CAD build for the part. Positions are in the model's coordinates, mm. A direction names the side the tool comes from. Round coordinates to 2 decimals unless told otherwise and drop trailing zeros. Loops run counter-clockwise (first coordinate to the right, second up) from the corner with the lowest first, then second, coordinate; pieces in that order, holes last. Notation, with made-up numbers: M 7,45 L 38,45 A20 ccw 38,69 Z; hole C 86,-26 d2. An arc over 180 degrees is marked long. Use one line per item in the form item = value.
Autodesk Inventor part; units mm, degrees
ref_plane "Work Plane3" through (-33.4299, 11.4299, 16.4) normal (0, 0, -1) x (0, 1, 0)
ref_plane "YZ Plane" through (0, 0, 0) normal (1, 0, 0) x (0, 1, 0)
ref_plane "XZ Plane" through (0, 0, 0) normal (0, 1, 0) x (-1, 0, 0)
ref_plane "Work Plane1" through (0, 0, 10) normal (0, 0, 1) x (1, 0, 0)
sketch "Sketch1" plane through (0, 0, 10) normal (0, 0, 1) x (1, 0, 0)
  line L0 (-4.0299, -0.3538) -> (-2.2322, 1.4439) construction
  arc A0 (-1.4439, 2.2322) -> (-2.2322, 1.4439) centre (-0.9299, 0.9299) ccw construction
  line L1 (-1.4439, 2.2322) -> (0.3538, 4.0299) construction
  line L2 (-37.8299, 42.2137) -> (-37.8299, 45.8299) construction
  line L3 (-37.8299, 45.8299) -> (-4.0299, 45.8299) construction
  line L4 (-4.0299, 45.8299) -> (-4.0299, 42.2137) construction
  line L5 (-4.0299, 4.0299) -> (0.3538, 4.0299)
  circle A1 centre (-20.9299, 20.9299) radius 17.5
  line L6 (-20.9299, 58.9723) -> (17.1124, 20.9299) construction
  line L7 (17.1124, 20.9299) -> (-20.9299, -17.1124) construction
  line L8 (-20.9299, -17.1124) -> (-58.9723, 20.9299) construction
  line L9 (-58.9723, 20.9299) -> (-20.9299, 58.9723) construction
  line L10 (-20.9299, 58.9723) -> (-20.9299, -17.1124) construction
  line L11 (17.1124, 20.9299) -> (-58.9723, 20.9299) construction
  line L12 (-20.9299, 58.9723) -> (32.8701, 58.9723) construction
  line L13 (-43.4299, 43.4299) -> (1.5701, 43.4299) construction
  line L14 (1.5701, 43.4299) -> (1.5701, -1.5701) construction
  line L15 (1.5701, -1.5701) -> (-43.4299, -1.5701) construction
  line L16 (-43.4299, -1.5701) -> (-43.4299, 43.4299) construction
  line L17 (-43.4299, 43.4299) -> (1.5701, -1.5701) construction
  line L18 (1.5701, 43.4299) -> (-43.4299, -1.5701) construction
  line L19 (-43.4299, 5.3876) -> (-43.4299, 36.4723)
  line L20 (-43.4299, 36.4723) -> (-36.4723, 43.4299)
  line L21 (-36.4723, 43.4299) -> (-5.3876, 43.4299)
  line L22 (-5.3876, 43.4299) -> (1.5701, 36.4723)
  line L23 (1.5701, 36.4723) -> (1.5701, 5.3876)
  line L24 (1.5701, 5.3876) -> (-5.3876, -1.5701)
  line L25 (-5.3876, -1.5701) -> (-36.4723, -1.5701)
  line L26 (-36.4723, -1.5701) -> (-43.4299, 5.3876)
  line L27 (-4.0299, 42.2137) -> (-37.8299, 42.2137)
  line L28 (-4.0299, -0.3538) -> (-4.0299, 4.0299)
  circle A2 centre (-20.9299, 20.9299) radius 7.0417
  point P0 (-37.8299, 4.0299)
  dimension "d18" = 53.8
  dimension "d19" = 45
  dimension "d20" = 53.8
  dimension "d21" = 45
  dimension "d22" = 45
extrude "Extrusion1" add sketch "Sketch1" along normal blind 3 contours L28 L24 L25 L26 L19 L20 L27 L22 L23 L5 | L5 L24 L28 | L27 L20 L21 L22 | A1
sketch "Sketch3" plane through (0, 0, 10) normal (0, 0, -1) x (-1, 0, 0)
  line L0 (37.8299, -0.4701) -> (37.8299, 4.0299) construction
  line L1 (4.0299, 4.0299) -> (4.0299, -0.4701) construction
  line L2 (37.8299, -0.4701) -> (37.8299, 1.1886) construction
  line L3 (4.0299, -3.9701) -> (4.0299, -0.3538) construction
  line L4 (45.8299, 4.0299) -> (42.2137, 4.0299) construction
  line L5 (-0.3538, 4.0299) -> (-3.9701, 4.0299) construction
  line L6 (-3.9701, 37.8299) -> (-0.3538, 37.8299) construction
  line L7 (4.0299, 42.2137) -> (4.0299, 45.8299) construction
  line L8 (37.8299, 45.8299) -> (37.8299, 42.2137) construction
  line L9 (42.2137, 37.8299) -> (45.8299, 37.8299) construction
  line L10 (37.8299, 37.7299) -> (45.8299, 37.7299)
  line L11 (45.8299, 37.7299) -> (45.8299, 4.1299)
  line L12 (45.8299, 4.1299) -> (37.8299, 4.1299)
  line L13 (37.8299, 4.1299) -> (37.8299, 37.7299)
  line L14 (37.7299, 4.0299) -> (4.1299, 4.0299)
  line L15 (4.1299, 4.0299) -> (4.1299, -3.9701)
  line L16 (4.1299, -3.9701) -> (37.7299, -3.9701)
  line L17 (37.7299, -3.9701) -> (37.7299, 4.0299)
  line L18 (4.0299, 4.1299) -> (-3.9701, 4.1299)
  line L19 (-3.9701, 4.1299) -> (-3.9701, 37.7299)
  line L20 (-3.9701, 37.7299) -> (4.0299, 37.7299)
  line L21 (4.0299, 37.7299) -> (4.0299, 4.1299)
  line L22 (4.1299, 37.8299) -> (37.7299, 37.8299)
  line L23 (37.7299, 37.8299) -> (37.7299, 45.8299)
  line L24 (37.7299, 45.8299) -> (4.1299, 45.8299)
  line L25 (4.1299, 45.8299) -> (4.1299, 37.8299)
  point P0 (0, 0)
  dimension "d23" = 0.1
  dimension "d24" = 0.1
  dimension "d25" = 0.1
  dimension "d26" = 0.1
  dimension "d27" = 0.1
extrude "Extrusion3" add sketch "Sketch3" against normal up to surface (3 mm away)
sketch "Sketch4" plane through (0, 0, 13) normal (0, 0, 1) x (1, 0, 0)
  line L0 (-33.4299, 35.4299) -> (-33.4299, 11.4299) construction
  line L1 (-33.4299, 11.4299) -> (-8.4299, 11.4299) construction
  line L2 (-8.4299, 11.4299) -> (-8.4299, 35.4299) construction
  line L3 (-8.4299, 35.4299) -> (-33.4299, 35.4299) construction
  circle A0 centre (-10.4299, 33.4299) radius 1.05 construction
  circle A1 centre (-10.4299, 20.9299) radius 1.05 construction
  circle A2 centre (-31.4299, 20.9299) radius 1.05 construction
  circle A3 centre (-31.4299, 33.4299) radius 1.05 construction
  line L4 (-15.4299, 29.8299) -> (-12.4299, 29.8299) construction
  line L5 (-15.4299, 31.8299) -> (-15.4299, 29.8299) construction
  line L6 (-12.4299, 31.8299) -> (-15.4299, 31.8299) construction
  line L7 (-12.4299, 29.8299) -> (-12.4299, 31.8299) construction
  line L8 (-8.4299, 35.4299) -> (-11.9299, 35.4299)
  line L9 (-11.9299, 35.4299) -> (-11.9299, 19.4299)
  line L10 (-11.9299, 19.4299) -> (-8.4299, 19.4299)
  line L11 (-8.4299, 19.4299) -> (-8.4299, 35.4299)
  line L12 (-33.4299, 35.4299) -> (-29.9299, 35.4299)
  line L13 (-29.9299, 35.4299) -> (-29.9299, 19.4299)
  line L14 (-29.9299, 19.4299) -> (-33.4299, 19.4299)
  line L15 (-33.4299, 19.4299) -> (-33.4299, 35.4299)
  line L16 (-33.4299, 35.4299) -> (-37.4299, 35.4299)
  line L17 (-37.4299, 35.4299) -> (-37.4299, 19.4299)
  line L18 (-37.4299, 19.4299) -> (-33.4299, 19.4299)
  line L19 (-33.4299, 19.4299) -> (-33.4299, 35.4299)
  line L20 (-8.4299, 35.4299) -> (-4.4299, 35.4299)
  line L21 (-4.4299, 35.4299) -> (-4.4299, 19.4299)
  line L22 (-4.4299, 19.4299) -> (-8.4299, 19.4299)
  line L23 (-8.4299, 19.4299) -> (-8.4299, 35.4299)
  point P0 (0, 0)
  dimension "d30" = 3.5
  dimension "d31" = 16
  dimension "d32" = 3.5
  dimension "d37" = 4
  dimension "d38" = 4
ref_plane "Work Plane3" through (-33.4299, 11.4299, 16.4) normal (0, 0, -1) x (0, 1, 0)
extrude "Extrusion4" add sketch "Sketch4" along normal up to surface (3.4 mm away)
sketch "Sketch5" plane through (-11.9299, 35.4299, 16.4) normal (0, 0, 1) x (1, 0, 0)
  circle A0 centre (1.5, -14.5) radius 1.05
  circle A1 centre (1.5, -2) radius 1.05
  circle A2 centre (-19.5, -2) radius 1.05
  circle A3 centre (-19.5, -14.5) radius 1.05
  point P0 (11.9299, -35.4299)
extrude "Extrusion5" cut sketch "Sketch5" against normal through all
sketch "Sketch7" plane through (-37.4299, 35.4299, 13) normal (0, 1, 0) x (1, 0, 0)
  line L0 (4.95, -3.4) -> (4.95, 3)
  line L1 (7.5, -3.4) -> (0, -3.4)
  line L2 (7.5, 0) -> (7.5, -3.4)
  line L3 (0, 0) -> (7.5, 0)
  line L4 (0, 0) -> (0, -3.4)
  line L5 (33, -3.4) -> (25.5, -3.4)
  line L6 (33, 0) -> (33, -3.4)
  line L7 (25.5, 0) -> (33, 0)
  line L8 (25.5, 0) -> (25.5, -3.4)
  line L9 (0, -3.4) -> (7.5, -3.4)
  line L10 (0, -3.4) -> (3, -3.4)
  line L11 (3, -3.4) -> (3, -13.4)
  line L12 (3, -13.4) -> (0, -13.4)
  line L13 (0, -13.4) -> (0, -3.4)
  line L14 (33, -3.4) -> (30, -3.4)
  line L15 (30, -3.4) -> (30, -13.4)
  line L16 (30, -13.4) -> (33, -13.4)
  line L17 (33, -13.4) -> (33, -3.4)
  line L18 (0, -13.4) -> (7, -13.4)
  line L19 (7, -13.4) -> (7, -15.4)
  line L20 (7, -15.4) -> (0, -15.4)
  line L21 (0, -15.4) -> (0, -13.4)
  line L22 (33, -13.4) -> (26, -13.4)
  line L23 (26, -13.4) -> (26, -15.4)
  line L24 (26, -15.4) -> (33, -15.4)
  line L25 (33, -15.4) -> (33, -13.4)
  line L26 (3, -12) -> (5, -12)
  line L27 (5, -12) -> (5, -10)
  line L28 (5, -10) -> (3, -10)
  line L29 (3, -10) -> (3, -12)
  line L30 (30, -12) -> (28, -12)
  line L31 (28, -12) -> (28, -10)
  line L32 (28, -10) -> (30, -10)
  line L33 (30, -10) -> (30, -12)
  line L34 (5, -10) -> (3, -8)
  line L35 (5, -10) -> (7.8284, -10) construction
  line L36 (28, -10) -> (30, -8)
  line L37 (0, -15.4) -> (-2.7154, 0)
  line L38 (-4.7423, 0) -> (-0.3, 0)
  line L39 (0, -15.4) -> (15.6376, -15.4) construction
  line L40 (-2.7154, 0) -> (0, 0)
  line L41 (0, -15.4) -> (0, 0)
  line L42 (33, -15.4) -> (35.7154, 0)
  line L43 (33, -15.4) -> (48.6376, -15.4) construction
  line L44 (35.7154, 0) -> (33, 0)
  line L45 (37.7423, 0) -> (33.3, 0)
  line L46 (33, -15.4) -> (33, 0)
  point P0 (37.4299, 13)
  dimension "d39" = 3
  dimension "d40" = 10
  dimension "d41" = 3
  dimension "d42" = 7
  dimension "d43" = 2
  dimension "d44" = 7
  dimension "d47" = 27
  dimension "d48" = 1.4
  dimension "d49" = 2
  dimension "d50" = 2
  dimension "d51" = 2
  dimension "d52" = 135
  dimension "d53" = 100
  dimension "d54" = 80
extrude "Extrusion6" add sketch "Sketch7" against normal up to surface (16 mm away) contours L11 L12 L13 L1 | L4 L13 L21 L37 L38 L40 | L34 L28 L11 | L12 L18 L19 L20 L21 | L28 L27 L26 L11 | L17 L16 L15 L5 | L6 L44 L42 L25 L17 | L25 L24 L23 L22 L16 | L15 L32 L36 | L15 L30 L31 L32
sketch "Sketch8" plane through (-29.9299, 35.4299, 16.4) normal (0, 1, 0) x (1, 0, 0)
  line L0 (0, 0) -> (-4.5, 0)
  line L1 (0, 3.4) -> (0, 0)
  line L2 (-10.2154, 3.4) -> (0, 3.4)
  line L3 (-10.2154, 3.4) -> (-7.5, -12)
  line L4 (-7.5, -12) -> (-0.5, -12)
  line L5 (-0.5, -12) -> (-0.5, -10)
  line L6 (-0.5, -10) -> (-4.5, -10)
  line L7 (-4.5, -10) -> (-4.5, -8.6)
  line L8 (-4.5, -8.6) -> (-2.5, -8.6)
  line L9 (-2.5, -8.6) -> (-2.5, -6.6)
  line L10 (-2.5, -6.6) -> (-4.5, -4.6)
  line L11 (-4.5, -4.6) -> (-4.5, 0)
  line L12 (18, 3.4) -> (28.2154, 3.4)
  line L13 (18, 3.4) -> (18, 0)
  line L14 (22.5, 0) -> (18, 0)
  line L15 (22.5, 0) -> (22.5, -4.6)
  line L16 (22.5, -4.6) -> (20.5, -6.6)
  line L17 (20.5, -6.6) -> (20.5, -8.6)
  line L18 (20.5, -8.6) -> (22.5, -8.6)
  line L19 (22.5, -8.6) -> (22.5, -10)
  line L20 (22.5, -10) -> (18.5, -10)
  line L21 (18.5, -10) -> (18.5, -12)
  line L22 (18.5, -12) -> (25.5, -12)
  line L23 (25.5, -12) -> (28.2154, 3.4)
  point P0 (29.9299, 16.4)
extrude "Extrusion7" add sketch "Sketch8" along normal up to surface (10.4 mm away)
sketch "Sketch9" plane through (-37.7299, 45.8299, 13) normal (0, 0, -1) x (-1, 0, 0)
  line L0 (0, -3.6577) -> (2.4154, -6.0731)
  line L1 (2.4154, -6.0731) -> (2.4154, 0)
  line L2 (2.4154, 0) -> (0, 0)
  line L3 (0, -3.6577) -> (0, 0)
  line L4 (-33.6, 0) -> (-33.6, -3.6577)
  line L5 (-33.6, 0) -> (-36.0154, 0)
  line L6 (-36.0154, -6.0731) -> (-36.0154, 0)
  line L7 (-36.0154, -6.0731) -> (-33.6, -3.6577)
  point P0 (-37.7299, -45.8299)
extrude "Extrusion8" cut sketch "Sketch9" against normal through all
sketch "Sketch10" plane through (-29.9299, 19.4299, 16.4) normal (0, 0, 1) x (1, 0, 0)
  line L0 (0, 26.4) -> (0, 0)
  line L1 (18, 0) -> (18, 26.4)
  line L2 (-3.3664, 3.2942) -> (21.6336, 3.2942)
  line L3 (21.6336, 3.2942) -> (21.6336, 11.2942)
  line L4 (21.6336, 11.2942) -> (-3.3664, 11.2942)
  line L5 (-3.3664, 11.2942) -> (-3.3664, 3.2942)
  line L6 (-3.3664, 3.2942) -> (21.6336, 11.2942) construction
  line L7 (21.6336, 3.2942) -> (-3.3664, 11.2942) construction
  point P0 (29.9299, -19.4299)
  point P1 (9.1336, 7.2942)
  dimension "d59" = 25
  dimension "d60" = 8
extrude "Extrusion9" cut sketch "Sketch10" against normal blind 1
sketch "Sketch11" plane through (-37.4299, 19.4299, 28.4) normal (0, 0, 1) x (1, 0, 0)
  line L0 (0, 0) -> (7, 0)
  line L1 (7, 0) -> (7, 26.4)
  line L2 (7, 26.4) -> (0, 26.4)
  line L3 (0, 26.4) -> (0, 0)
  line L4 (26, 0) -> (33, 0)
  line L5 (33, 0) -> (33, 26.4)
  line L6 (33, 26.4) -> (26, 26.4)
  line L7 (26, 0) -> (26, 26.4)
  circle A0 centre (16.5, 1.5) radius 7.0417
  circle A1 centre (6, 1.5) radius 1.05 construction
  circle A2 centre (6, 14) radius 1.05 construction
  line L8 (27, 1.5) -> (6, 1.5) construction
  line L9 (27, 4.6642) -> (6, 4.6642)
  line L10 (6, -1.6642) -> (27, -1.6642)
  arc A3 (27, -1.6642) -> (27, 4.6642) centre (27, 1.5) ccw
  arc A4 (6, 4.6642) -> (6, -1.6642) centre (6, 1.5) ccw
  line L11 (27, 14) -> (6, 14) construction
  line L12 (27, 17.1642) -> (6, 17.1642)
  line L13 (6, 10.8358) -> (27, 10.8358)
  arc A5 (27, 10.8358) -> (27, 17.1642) centre (27, 14) ccw
  arc A6 (6, 17.1642) -> (6, 10.8358) centre (6, 14) ccw
  point P0 (37.4299, -19.4299)
  point P1 (16.5, 14)
extrude "Extrusion10" cut sketch "Sketch11" against normal blind 10 contours A4 L9 L1 L0 | L0 L1 L9 A0 L10 A4 | A0 L9 L10 | L12 L7 L13 L1 | L1 L13 A6 L12 | A0 L9 L7 L4 A3 L10 | L12 A5 L13 L7 | L9 A3 L4 L7
properties part number "50_Cube_Insert_Thorlabs"
1. Probe line 1 along Z through (x, y) = (1, 7); line 2 along X through (y, z) = (34.5, 21); line 3 along Y through (x, z) = (-35, 23.75). List the from-to ranges inside material, lowest first. Write a range as from..to.
Completed:
line_1 = 10..13
line_2 = -38.73..-34.43, -7.43..-3.13
line_3 = 19.43..45.83
2. Drop flat-ended pins along their axis: P1, Ø0.8, axis at y = 25, z = 16, coming from the +X side; P2, Ø8, axis at y = 12.5, z = 20.5, coming from the -X side; P3, Ø0.9, axis at x = -44.5, z = 11, coming from the -Y side; P4, Ø0.8, axis at x = -11, z = 27.5, coming from the -Y side. Give the stop position or say it passes through.
Completed:
P1 = -2.17
P2 = through
P3 = 4.13
P4 = 24.09
3. Cut at C-C on z = 19.5. Write the cut outline in (x, y), and give its area (3 significant figures).
Completed:
outline = M -39,19.43 L -34.43,19.43 L -34.43,19.92 A3.16 cw -34.43,21.94 L -34.43,32.42 A3.16 cw -34.43,34.44 L -34.43,45.83 L -37.73,45.83 L -37.73,42.17 L -39,40.9 Z; M -7.43,19.43 L -2.86,19.43 L -2.86,40.9 L -4.13,42.17 L -4.13,45.83 L -7.43,45.83 L -7.43,34.44 A3.16 cw -7.43,32.42 L -7.43,21.94 A3.16 cw -7.43,19.92 Z
area = 229 mm2
4. Cut at B-B on x = -16.5. Write the cut outline in (y, z), and give its area (3 significant figures).
Completed:
outline = M -3.97,10 L 15.46,10 L 15.46,13 L -3.97,13 Z; M 26.4,10 L 45.83,10 L 45.83,13 L 26.4,13 Z
area = 117 mm2
5. Tool access for faces 1 (the face through (2, 4.13, 11)), 2 (the face through (-9, 35, 16.4)), 3 (the face through (-37.73, 44, 18)), 4 (the face through (-32, 27, 15.4)): list every direction of +Z, -Z, +X, -X, +Y, -Y with a clear straight run to the whole face (end or side of a thin tool).
Completed:
face_1 = +Z, -Z, +X, -Y
face_2 = +Y, -Y
face_3 = +Z, -Z, -X, +Y
face_4 = none
6. Pull direction Z, two halves, no side cores. Call faces 5 (the face through (-7.43, 33, 18)), 6 (the face through (-3.09, 29.88, 20.81)), 7 (the face through (-40, 39.9, 11.5)): +Z half, -Z half, draft (parallel to the pull), parting line (faces both ways), or undercut.
Completed:
face_5 = undercut
face_6 = +Z half
face_7 = draft
7. Cut at A-A on z = 14.75. Write the cut outline in (x, y).
Completed:
outline = M -39.84,19.43 L -29.93,19.43 L -29.93,45.83 L -37.73,45.83 L -37.73,42.17 L -39.84,40.07 Z; M -11.93,19.43 L -2.02,19.43 L -2.02,40.07 L -4.13,42.17 L -4.13,45.83 L -11.93,45.83 Z; hole C -31.43,20.93 d2.1; hole C -31.43,33.43 d2.1; hole C -10.43,20.93 d2.1; hole C -10.43,33.43 d2.1
